The listing builds one solid part. Answer for the finished solid, in the listing's coordinates (mm). Give positions to 0.01 mm unless a question says otherwise; leave off trailing zeros. Write each loop counter-clockwise with the first axis right and the second up, starting at its lowest first coordinate (ties: lowest second). Pieces come first, ordered by that corner, then holes. Notation, with made-up numbers: (-21, 0) -> (-16, 0) arc R8 ccw to (-16, 9) -> close; hole circle Ø8 at (22, -36.5). An arc over 180 degrees is marked (long way). Put each result on its own line as item: value. Start each with the question number.
1) A cutting plane is placed at A-A (x = 20). Write down the section's boundary in (y, z).
2) Find the intervals of material crossed by line 1 along X through (y, z) = (-72, 0.9); line 2 along X through (y, z) = (72, 2.25); line 3 along Y through (x, z) = (30.26, 1.05), in increasing order. Write a range as from..to.
3) For a pull along X with two mould halves and no side action, classify faces 1 (the cylindrical face through (-22.05, 0.09, 1.52)), 2 (the cylindrical face through (-56.96, -57.55, 1.48)), 3 (the flat face through (-1, 1, 0)) as released by +X, released by -X, zero draft, split by the parting line, or undercut.
from build123d import *

# Parameters (mm, degrees)
SKETCH1_W           = 150
SKETCH1_H           = 150
BOSS_EXTRUDE1_DEPTH = 3
FILLET1_R           = 3
SKETCH2_R           = 2.1
CUT_EXTRUDE1_DEPTH  = 3
SKETCH3_R           = 1
CUT_EXTRUDE2_DEPTH  = 3
CUT_EXTRUDE_1_REACH = 108.108
SKETCH_2_R          = 2.05


with BuildPart() as part:
    # Sketch1 → Boss-Extrude1 (new body)
    with BuildSketch(Plane.XY):
        Rectangle(SKETCH1_W, SKETCH1_H)
    extrude(amount=BOSS_EXTRUDE1_DEPTH)

    # Fillet1
    fillet1_edges = [part.edges().sort_by_distance(p)[0] for p in [
        (75, -75, 1.5),
        (-75, -75, 1.5),
        (-75, 75, 1.5),
        (75, 75, 1.5),
    ]]
    fillet(fillet1_edges, radius=FILLET1_R)

    # Sketch2 → Cut-Extrude1 (cut)
    with BuildSketch(Plane(origin=(0, 0, 0), x_dir=(-1, 0, 0), z_dir=(0, 0, -1))):
        with Locations((-55.835, 59.325)):
            Circle(SKETCH2_R)
        with Locations((55.835, 59.325)):
            Circle(SKETCH2_R)
        with Locations((-55.835, -59.325)):
            Circle(SKETCH2_R)
        with Locations((55.835, -59.325)):
            Circle(SKETCH2_R)
    extrude(amount=-CUT_EXTRUDE1_DEPTH, mode=Mode.SUBTRACT)

    # Sketch3 → Cut-Extrude2 (cut)
    with BuildSketch(Plane(origin=(0, 0, 0), x_dir=(-1, 0, 0), z_dir=(0, 0, -1))):
        with Locations((-52.26, 72)):
            Circle(SKETCH3_R)
        with Locations((-30.26, 72)):
            Circle(SKETCH3_R)
        with Locations((52.26, -72)):
            Circle(SKETCH3_R)
        with Locations((30.26, -72)):
            Circle(SKETCH3_R)
    extrude(amount=-CUT_EXTRUDE2_DEPTH, mode=Mode.SUBTRACT)

    # 草图2 → 切除-拉伸1 (cut, up to next)
    with BuildSketch(Plane.XY.offset(3), mode=Mode.PRIVATE) as cut_extrude_1_sk1:
        with Locations((-30, 0)):
            Circle(SKETCH_2_R)
    cut_extrude_1_tool1 = extrude(cut_extrude_1_sk1.sketch, amount=-CUT_EXTRUDE_1_REACH, mode=Mode.PRIVATE) & part.part
    # 草图2 → 切除-拉伸1 (cut, up to next)
    with BuildSketch(Plane.XY.offset(3), mode=Mode.PRIVATE) as cut_extrude_1_sk2:
        with Locations((-20, 0)):
            Circle(SKETCH_2_R)
    cut_extrude_1_tool2 = extrude(cut_extrude_1_sk2.sketch, amount=-CUT_EXTRUDE_1_REACH, mode=Mode.PRIVATE) & part.part
    # 草图2 → 切除-拉伸1 (cut, up to next)
    with BuildSketch(Plane.XY.offset(3), mode=Mode.PRIVATE) as cut_extrude_1_sk3:
        with Locations((30, 0)):
            Circle(SKETCH_2_R)
    cut_extrude_1_tool3 = extrude(cut_extrude_1_sk3.sketch, amount=-CUT_EXTRUDE_1_REACH, mode=Mode.PRIVATE) & part.part
    # 草图2 → 切除-拉伸1 (cut, up to next)
    with BuildSketch(Plane.XY.offset(3), mode=Mode.PRIVATE) as cut_extrude_1_sk4:
        with Locations((20, 0)):
            Circle(SKETCH_2_R)
    cut_extrude_1_tool4 = extrude(cut_extrude_1_sk4.sketch, amount=-CUT_EXTRUDE_1_REACH, mode=Mode.PRIVATE) & part.part
    add(cut_extrude_1_tool1.solids().sort_by_distance((-30, 0, 3))[0], mode=Mode.SUBTRACT)
    add(cut_extrude_1_tool2.solids().sort_by_distance((-20, 0, 3))[0], mode=Mode.SUBTRACT)
    add(cut_extrude_1_tool3.solids().sort_by_distance((30, 0, 3))[0], mode=Mode.SUBTRACT)
    add(cut_extrude_1_tool4.solids().sort_by_distance((20, 0, 3))[0], mode=Mode.SUBTRACT)


solid = part.part
Reply:
1. outline: (-75, 0) -> (-2.05, 0) -> (-2.05, 3) -> (-75, 3) -> close; (2.05, 0) -> (75, 0) -> (75, 3) -> (2.05, 3) -> close
2. line 1: x = -75..-53.26, -51.26..-31.26, -29.26..75
2. line 2: x = -75..29.26, 31.26..51.26, 53.26..75
2. line 3: y = -75..-2.03, 2.03..71, 73..75
3. face 1: undercut
3. face 2: undercut
3. face 3: zero draft
